Check sheet for the drawn part. Datum: minimum x, y, z corner. Units: mm. A direction names the side the tool comes from. Give positions to 0.01 mm unless a question says otherwise; leave off trailing zeros. Loops run counter-clockwise (first coordinate to the right, second up) from the corner with the lowest first, then second, coordinate; pieces in that order, holes last. Notation, with made-up numbers: (70.25, 35.5) - (124.25, 35.5) arc R30 cw to (124.25, 63.5) - close; hole circle Ø7 at (25, 82.25). An arc over 180 degrees is marked (long way). Use a Markdown table: item, result. Add a question column.
1. Cross-section at B-B on y = 63.5. Enter the section's corners in (x, z) (3 decimals), and give its area (3 significant figures).
2. Cross-section at D-D on y = 26. Enter the section's corners in (x, z) (3 decimals), and give its area (3 significant figures).
3. Set-up check for the marked faces 4 and 5: record each of +Z, -Z, +X, -X, +Y, -Y from which the full face is reachable in a straight line by a thin tool's end or side.
4. Depth check by flat-ended pin: P1, Ø7.5, axis at x = 314.5, y = 53.5, coming from the -Z side (3 decimals); P2, Ø1.5, axis at y = 47.5, z = 18.5, coming from the +X side; P3, Ø5, axis at x = 141, y = 35, coming from the -Z side. Enter the tip coordinate at first touch or a pass-through.
5. Cross-section at C-C on z = 59.5. Enter the section's corners in (x, y).
6. Draft check along X on the marked faces 1, 2 and 3. Enter one of: pulls with the +X half, pulls with the -X half, needs draft (parallel to the pull), parting line crosses it, or undercut.
7. Material ranges on L1, parallel to Y at x = 12.7, z = 127 (3 decimals); L2, parallel to X at y = 63, z = 125; L3, parallel to X at y = 32, z = 39.5 (1 decimal), recorded low to high.
8. Cross-section at A-A on x = 12.7. Enter the section's corners in (y, z) (3 decimals), and give its area (3 significant figures).
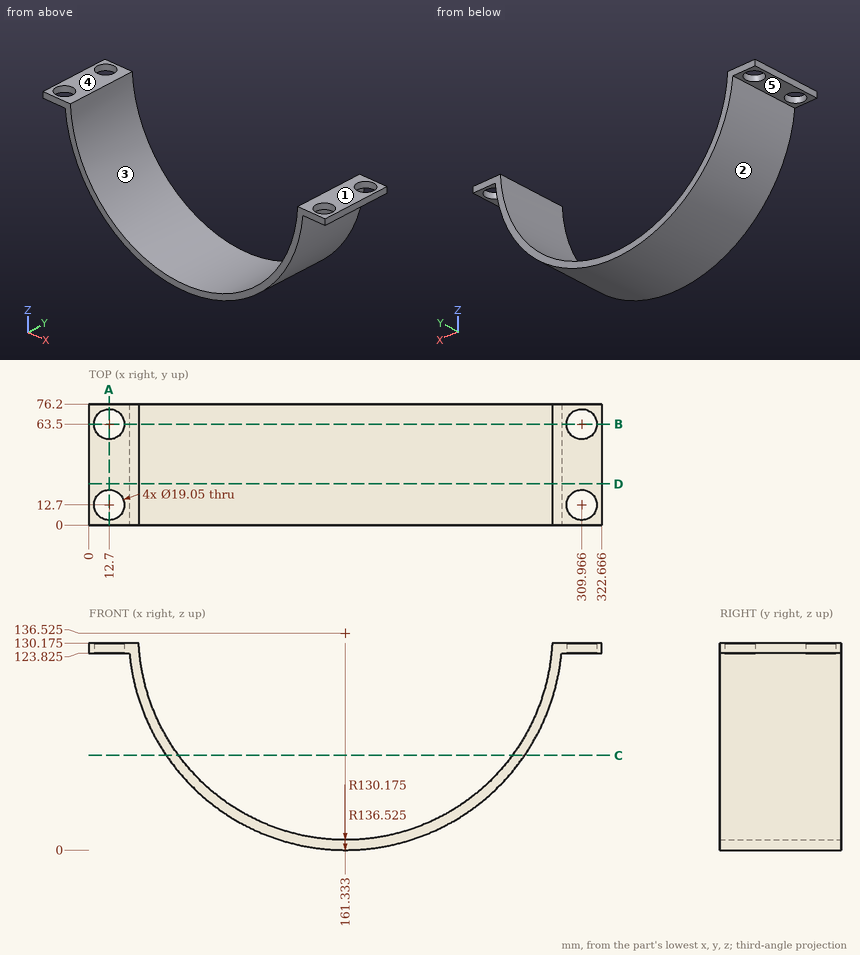
Values found:
| question | item | result |
|---|---|---|
| 1 | outline | (0, 123.825) - (3.175, 123.825) - (3.175, 130.175) - (0, 130.175) - close; (22.225, 123.825) - (25.4, 123.825) arc R136.525 ccw to (297.266, 123.825) - (300.441, 123.825) - (300.441, 130.175) - (291.353, 130.175) arc R130.175 cw to (31.313, 130.175) - (22.225, 130.175) - close; (319.491, 123.825) - (322.666, 123.825) - (322.666, 130.175) - (319.491, 130.175) - close |
| 1 | area | 2,660 mm2 |
| 2 | outline | (0, 123.825) - (25.4, 123.825) arc R136.525 ccw to (297.266, 123.825) - (322.666, 123.825) - (322.666, 130.175) - (291.353, 130.175) arc R130.175 cw to (31.313, 130.175) - (0, 130.175) - close |
| 2 | area | 2,900 mm2 |
| 3 | face 4 | +Z, +X, -X, +Y, -Y |
| 3 | face 5 | -Z, -X, +Y, -Y |
| 4 | P1 | stops at z = 123.825 |
| 4 | P2 | stops at x = 231.23 |
| 4 | P3 | stops at z = 1.17 |
| 5 | outline | (48.61, 0) - (56.39, 0) - (56.39, 76.2) - (48.61, 76.2) - close; (266.27, 0) - (274.05, 0) - (274.05, 76.2) - (266.27, 76.2) - close |
| 6 | face 1 | needs draft |
| 6 | face 2 | parting line crosses it |
| 6 | face 3 | undercut |
| 7 | L1 | y = 0 to 3.175, 22.225 to 53.975, 73.025 to 76.2 |
| 7 | L2 | x = 0 to 3.19, 22.21 to 31.67, 291 to 300.45, 319.48 to 322.67 |
| 7 | L3 | x = 65.3 to 74.5, 248.1 to 257.4 |
| 8 | outline | (0, 123.825) - (3.175, 123.825) - (3.175, 130.175) - (0, 130.175) - close; (22.225, 123.825) - (53.975, 123.825) - (53.975, 130.175) - (22.225, 130.175) - close; (73.025, 123.825) - (76.2, 123.825) - (76.2, 130.175) - (73.025, 130.175) - close |
| 8 | area | 242 mm2 |
